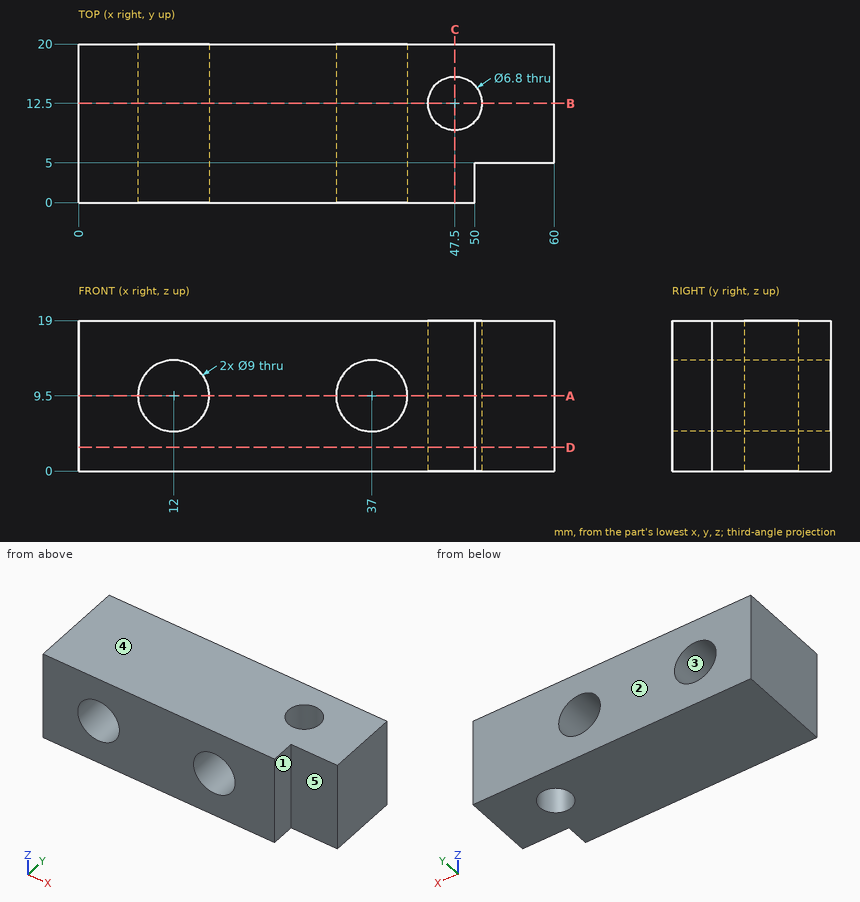
Input: dimensioned drawing with shaded views. Units: mm. Origin: part minimum x, y, z. A direction names the side the tool comes from. Give positions to 0.01 mm unless a question says otherwise; leave off trailing zeros. Write each loop counter-clockwise with the first axis right and the second up, starting at its lowest first coordinate (ties: lowest second). Pieces come first, ordered by that corner, then holes.
Q1. Section D-D, the plane z = 3. Output: boundary loops of the cut face in (x, y).
Q2. Material intervals for probe 1 along X at (y, z) = (6, 9.25); probe 2 along Y at (x, z) = (47.5, 4.5); probe 3 along X at (y, z) = (1.5, 8.5), sorted ascending.
Q3. Set-up query: the marked faces 4 and 5. Return all of +Z, -Z, +X, -X, +Y, -Y with unobstructed straight access to the full face (end or side cutting, diameter ignored); none if empty.
Q4. Pull-direction query (X, two-part tool) for the marked faces 1, 2 and 3; classes: pulls with the +X half, pulls with the -X half, needs draft (parallel to the pull), parting line crosses it, or undercut.
Q5. Section C-C, the plane x = 47.5. Output: boundary loops of the cut face in (y, z), plus the area to 3 significant figures.
Q6. Section A-A, the plane z = 9.5. Output: boundary loops of the cut face in (x, y).
Q7. Section B-B, the plane y = 12.5. Output: boundary loops of the cut face in (x, z).
Q8. First-contact query: P1, Ø5.5, axis at x = 12, z = 9.5, coming from the -Y side; P2, Ø1, axis at y = 13, z = 4, coming from the -X side; P3, Ø2.5, axis at y = 2, z = 12.5, coming from the +X side. Flat tips, straight axial feed; report the tip coordinate or a pass-through.
Filled in:
1. outline: (0, 0) - (50, 0) - (50, 5) - (60, 5) - (60, 20) - (0, 20) - close; hole circle Ø6.8 at (47.5, 12.5)
2. probe 1: x = 0 to 7.51, 16.49 to 32.51, 41.49 to 60
2. probe 2: y = 0 to 9.1, 15.9 to 20
2. probe 3: x = 0 to 7.61, 16.39 to 32.61, 41.39 to 50
3. face 4: +Z, +X, -X, +Y, -Y
3. face 5: +Z, -Z, +X, -Y
4. face 1: pulls with the +X half
4. face 2: needs draft
4. face 3: undercut
5. outline: (0, 0) - (9.1, 0) - (9.1, 19) - (0, 19) - close; (15.9, 0) - (20, 0) - (20, 19) - (15.9, 19) - close
5. area: 251 mm2
6. outline: (0, 0) - (7.5, 0) - (7.5, 20) - (0, 20) - close; (16.5, 0) - (32.5, 0) - (32.5, 20) - (16.5, 20) - close; (41.5, 0) - (50, 0) - (50, 5) - (60, 5) - (60, 20) - (41.5, 20) - close; hole circle Ø6.8 at (47.5, 12.5)
7. outline: (0, 0) - (44.1, 0) - (44.1, 19) - (0, 19) - close; (50.9, 0) - (60, 0) - (60, 19) - (50.9, 19) - close; hole circle Ø9 at (12, 9.5); hole circle Ø9 at (37, 9.5)
8. P1: passes through
8. P2: stops at x = 0
8. P3: stops at x = 50
